```python
from build123d import *

# Parameters (mm, degrees)
F3_DEPTH = 1.27
F4_R     = 0.3175
F5_DEPTH = 44.2922501


# Not quite as in the source:
# - the dataset's text gives a spline's control points without its knots; the knots are read off the source's solid


with BuildPart() as f1:
    # F0 (on Right) → F1 (revolve)
    with BuildSketch(Plane.YZ):
        with BuildLine():
            Line((0, 34.13125), (0, 31.75))
            add(Edge.make_bspline(
                [(0, 31.75), (0.5742670905, 30.3542906008), (2.3414834837, 25.8865164681), (3.175, 10.5516560434), (3.175, 0)],
                knots=[0, 0, 0, 0, 0.3124675666, 1, 1, 1, 1], degree=3))
            Line((3.175, 0), (5.55625, 0))
            add(Edge.make_bspline(
                [(2.2021322713, 32.6560712016), (2.3186413793, 32.3729053021), (2.5576698716, 31.7878917938), (2.9240965193, 30.812098832), (3.2829237449, 29.7062776723), (3.6213582396, 28.4414870624), (3.9333609229, 26.9775001767), (4.2135585587, 25.2856930459), (4.4651056247, 23.3880591837), (4.7658122637, 20.5979082433), (5.0781689931, 16.6702210435), (5.3509257758, 11.4172981506), (5.5180630854, 5.8010058197), (5.55625, 1.9340677683), (5.55625, 0)],
                knots=[1e-10, 1e-10, 1e-10, 1e-10, 0.0625000001, 0.1250000001, 0.1875000001, 0.2500000001, 0.3125000001, 0.3750000001, 0.4375000001, 0.5, 0.625, 0.75, 0.875, 1, 1, 1, 1], degree=3))
            ThreePointArc((2.2021322713, 32.6560712016), (1.3252866697, 33.728374789), (0, 34.13125))
        make_face()
    revolve(axis=Axis((0, 4.365625, 0), (0, -1, 0)))

    # F2 (on face) → F3 (join)
    with BuildSketch(Plane.XZ):
        with BuildLine():
            Line((-10.16, -30.0805069771), (-10.16, -35.2621069771))
            Line((-10.16, -35.2621069771), (10.16, -35.2621069771))
            Line((10.16, -35.2621069771), (10.16, -30.0805069771))
            ThreePointArc((10.16, -30.0805069771), (0, -31.75), (-10.16, -30.0805069771))
        make_face()
    extrude(amount=-F3_DEPTH)

    # F4 (on face) → F5 (cut, through all)
    with BuildSketch(Plane.YZ.offset(10.16)):
        with Locations((0.635, -34.6159934103)):
            Circle(F4_R)
        with BuildLine():
            Line((1.27, -35.2621069771), (1.27, -34.6159934103))
            ThreePointArc((1.27, -34.6159934103), (0.635, -35.2509934103), (0, -34.6159934103))
            Line((0, -34.6159934103), (0, -35.2621069771))
            Line((0, -35.2621069771), (1.27, -35.2621069771))
        make_face()
    extrude(amount=-F5_DEPTH, mode=Mode.SUBTRACT)


solid = f1.part
```
CAD build for the part. Positions are in the model's coordinates, mm. A direction names the side the tool comes from. Coordinates: 2 decimals unless noted, no trailing zeros.
(1) Flat gauge pins, fed straight in: pin 1 (10 mm diameter, centred on x = -16, z = -8.5, fed in from +Y); pin 2 (2.5 mm diameter, centred on x = -2.5, z = -33, fed in from +Y); pin 3 (2 mm diameter, centred on x = -21.5, y = 3, fed in from -Z). Where does each tip first touch, or does it go through?
(2) 3-axis set-ups, long thin cutter, end or side, ignore diameter. For faces 1 (the face through (28, 0, -16)), 2 (the face through (0, 1.27, -34)): which of +Z, -Z, +X, -X, +Y, -Y reach the whole face in a straight line?
(3) Drill centre lines: probe 1 along Z at (x, y) = (30.5, 1.25); probe 2 along Y at (x, z) = (12, 0); probe 3 along Y at (x, z) = (14, -4). Where is each one in solid material? Low to high.
Geometry says:
1. pin 1: stops at y = 5.26
1. pin 2: stops at y = 2.53
1. pin 3: stops at z = -25.25
2. face 1: +Z, -Z, +X, -X, -Y
2. face 2: -Z, +Y
3. probe 1: z = -14.51 to 14.51
3. probe 2: y = 2.92 to 5.31
3. probe 3: y = 2.8 to 5.18
